The figure shows three views and two pictorial views of one solid part (mm, origin at its lowest corner). Answer the questions. A direction names the side the tool comes from. Round coordinates to 2 decimals unless told otherwise and drop trailing zeros. Order: outer loops, then holes, each group sorted by start corner. A loop starts at its lowest first (then second) coordinate and runs counter-clockwise, first axis right, second up. Notation, with made-up numbers: (34, -7) - (56, -7) arc R11 ccw to (56, 1) - close; hole circle Ø1 at (35.5, -0.5). An arc over 180 degrees is marked (long way). Write item = value, one per line.
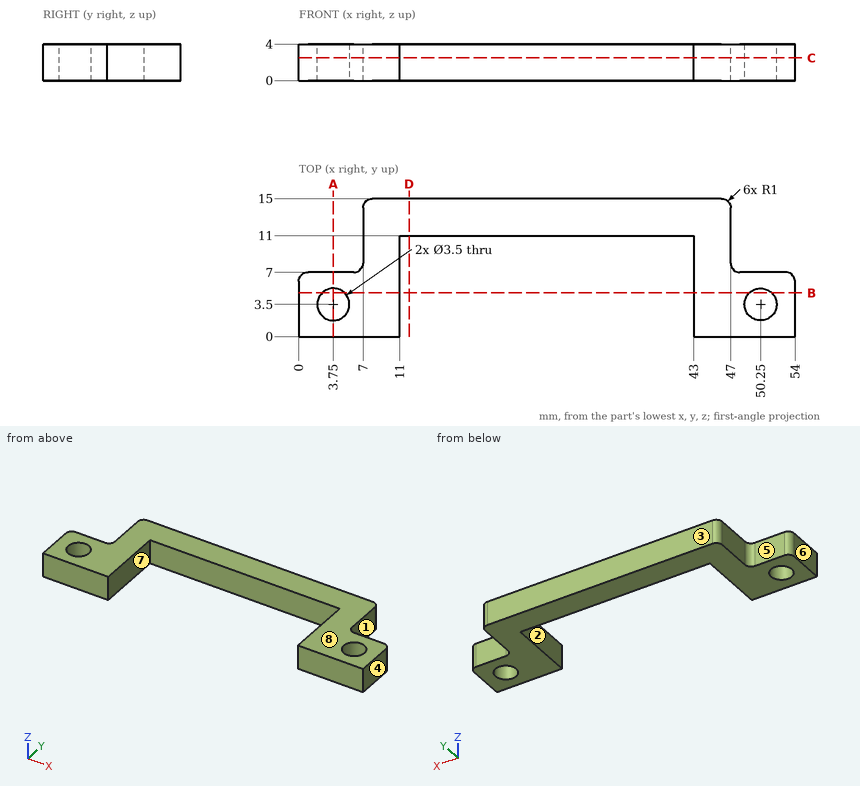
Q1. Section B-B on y = 4.75 is taken. Determine the outline of the cut face in (x, z).
Model answer:
outline = (0, 0) - (2.53, 0) - (2.53, 4) - (0, 4) - close; (4.97, 0) - (11, 0) - (11, 4) - (4.97, 4) - close; (43, 0) - (49.03, 0) - (49.03, 4) - (43, 4) - close; (51.47, 0) - (54, 0) - (54, 4) - (51.47, 4) - close
Q2. Find the intervals of material crossed by line 1 (Y direction, x = 3.75, z = 1.35); line 2 (X direction, y = 4, z = 3.5); line 3 (X direction, y = 13.75, z = 0.4), in increasing order. Write a range as from..to.
Model answer:
line_1 = 0..1.75, 5.25..7
line_2 = 0..2.07, 5.43..11, 43..48.57, 51.93..54
line_3 = 7..47
Q3. Flat-ended cylindrical pins translate along their axes: P1, Ø3, axis at x = 3.75, y = 3.5, coming from the +Z side; P2, Ø2, axis at x = 2.5, z = 1.5, coming from the +Y side; P3, Ø1.2, axis at x = 23.5, z = 3, coming from the -Y side. Find the tip coordinate at first contact, or state that the pin passes through.
Model answer:
P1 = through
P2 = 7
P3 = 11
Q4. Determine the mould class of the marked faces 6, 7 and 8 for opening direction X: released by +X, released by -X, zero draft, split by the parting line, or undercut.
Model answer:
face_6 = released by -X
face_7 = undercut
face_8 = zero draft
Q5. Section D-D on x = 12 is taken. Determine the outline of the cut face in (y, z).
Model answer:
outline = (11, 0) - (15, 0) - (15, 4) - (11, 4) - close
Q6. For the marked faces 1, 2, 3, 4 and 5, determine the directions among +Z, -Z, +X, -X, +Y, -Y from which every point of the face is accessible in a straight line to the end or side of a thin tool.
Model answer:
face_1 = +Z, -Z, +X, +Y
face_2 = +Z, -Z, -Y
face_3 = +Z, -Z, +X, -X, +Y
face_4 = +Z, -Z, +X, +Y, -Y
face_5 = +Z, -Z, -X, +Y
Q7. Section A-A on x = 3.75 is taken. Determine the outline of the cut face in (y, z), then the cut area to 3 significant figures.
Model answer:
outline = (0, 0) - (1.75, 0) - (1.75, 4) - (0, 4) - close; (5.25, 0) - (7, 0) - (7, 4) - (5.25, 4) - close
area = 14.0 mm^2
Q8. Section C-C on z = 2.5 is taken. Determine the outline of the cut face in (x, y).
Model answer:
outline = (0, 0) - (11, 0) - (11, 11) - (43, 11) - (43, 0) - (54, 0) - (54, 6) arc R1 ccw to (53, 7) - (48, 7) arc R1 cw to (47, 8) - (47, 14) arc R1 ccw to (46, 15) - (8, 15) arc R1 ccw to (7, 14) - (7, 8) arc R1 cw to (6, 7) - (1, 7) arc R1 ccw to (0, 6) - close; hole circle Ø3.5 at (3.75, 3.5); hole circle Ø3.5 at (50.25, 3.5)
